from build123d import *

# Parameters (mm, degrees)
SKETCH1_R           = 4
BOSS_EXTRUDE1_DEPTH = 40
SKETCH3_R           = 8
BOSS_EXTRUDE2_DEPTH = 20
SKETCH4_R           = 5
BOSS_EXTRUDE3_DEPTH = 108
SKETCH5_W           = 14
SKETCH5_H           = 2
BOSS_EXTRUDE4_DEPTH = 130
CUT_EXTRUDE1_REACH  = 26
SKETCH6_R           = 4


with BuildPart() as part:
    # Sketch1 → Boss-Extrude1 (new body, symmetric)
    with BuildSketch(Plane(origin=(0, 0, 0), x_dir=(1, 0, 0), z_dir=(0, 1, 0))):
        Circle(SKETCH1_R)
    extrude(amount=BOSS_EXTRUDE1_DEPTH, both=True)

    # Sketch3 → Boss-Extrude2 (add, symmetric)
    with BuildSketch(Plane(origin=(0, 0, 0), x_dir=(1, 0, 0), z_dir=(0, 1, 0))):
        Circle(SKETCH3_R)
    extrude(amount=BOSS_EXTRUDE2_DEPTH, both=True)

    # Sketch4 → Boss-Extrude3 (add)
    with BuildSketch(Plane(origin=(0, 0, 0), x_dir=(0, 0, -1), z_dir=(1, 0, 0))):
        Circle(SKETCH4_R)
    extrude(amount=BOSS_EXTRUDE3_DEPTH)

    # Sketch5 → Boss-Extrude4 (add)
    with BuildSketch(Plane.XY):
        with Locations((0, -17)):
            Rectangle(SKETCH5_W, SKETCH5_H)
    extrude(amount=BOSS_EXTRUDE4_DEPTH)

    # Sketch6 → Cut-Extrude1 (cut, up to next)
    with BuildSketch(Plane(origin=(0, -16, 0), x_dir=(1, 0, 0), z_dir=(0, 1, 0)), mode=Mode.PRIVATE) as cut_extrude1_sk1:
        with Locations((0, -120)):
            Circle(SKETCH6_R)
    cut_extrude1_tool1 = extrude(cut_extrude1_sk1.sketch, amount=-CUT_EXTRUDE1_REACH, mode=Mode.PRIVATE) & part.part
    add(cut_extrude1_tool1.solids().sort_by_distance((0, -16, 120))[0], mode=Mode.SUBTRACT)


solid = part.part
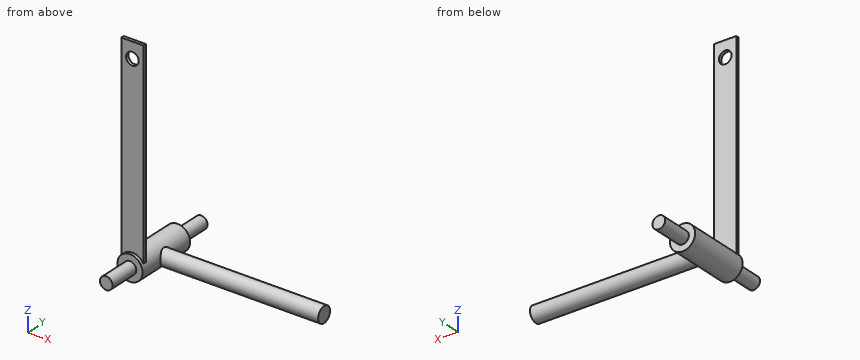
Here's how the part is built. I have some questions about the finished solid (model axes, mm). Round coordinates to 2 decimals unless told otherwise and drop trailing zeros. Order: outer loops, then holes, each group sorted by start corner. A loop starts at its lowest first (then second) coordinate and runs counter-clockwise, first axis right, second up. Notation, with made-up numbers: M 16,81 L 35,81 A21 cw 35,98 Z; hole C -38.75,38 d7. An arc over 180 degrees is marked long. Return JSON: item names as keys, results as strings. Group by question number.
1. I'm going to push flat-ended pins straight in: pin 1 Ø1 at (y, z) = (-17, 56.5) entering from +X; pin 2 Ø15.5 at (x, z) = (-3.5, 59) entering from +Y; pin 3 Ø10 at (x, y) = (4.5, 12.5) entering from +Z. Where does each tip first touch, or does it pass through?
2. If we section it at A-A on z = 120: List the corners of the cut face in (x, y) for me.
3. If we section it at B-B on x = 0: List the corners of the cut face in (y, z) for me, then the cut area to 3 significant figures.
4. If we section it at D-D on y = 0: List the corners of the cut face in (x, z) for me (3 decimals), then the cut area to 3 significant figures.
5. Please list where these lines run through material, in increasing order: probe 1 along X at (y, z) = (-17.15, 120); probe 2 along Z at (x, y) = (0, -17); probe 3 along Z at (x, y) = (-1.5, -7).
6. If we section it at C-C on z = 0: List the corners of the cut face in (x, y) for me.
Reply:
{
 "1": {"pin 1": "x = 7", "pin 2": "y = -16", "pin 3": "z = 8"},
 "2": {"outline": "M -7,-18 L -4,-18 L -4,-16 L -7,-16 Z; M 4,-18 L 7,-18 L 7,-16 L 4,-16 Z"},
 "3": {"outline": "M -40,-4 L -20,-4 L -20,-8 L 20,-8 L 20,-4 L 40,-4 L 40,4 L 20,4 L 20,8 L -16,8 L -16,116 L -18,116 L -18,8 L -20,8 L -20,4 L -40,4 Z; M -18,124 L -16,124 L -16,130 L -18,130 Z", "area": "1,190 mm^2"},
 "4": {"outline": "M 6.245,-5 L 108,-5 L 108,5 L 6.245,5 A8 ccw long Z", "area": "1,210 mm^2"},
 "5": {"probe 1": "-7 to -4, 4 to 7", "probe 2": "-8 to 116, 124 to 130", "probe 3": "-7.86 to 7.86"},
 "6": {"outline": "M -8,-20 L -4,-20 L -4,-40 L 4,-40 L 4,-20 L 8,-20 L 8,-5 L 108,-5 L 108,5 L 8,5 L 8,20 L 4,20 L 4,40 L -4,40 L -4,20 L -8,20 Z"}
}
